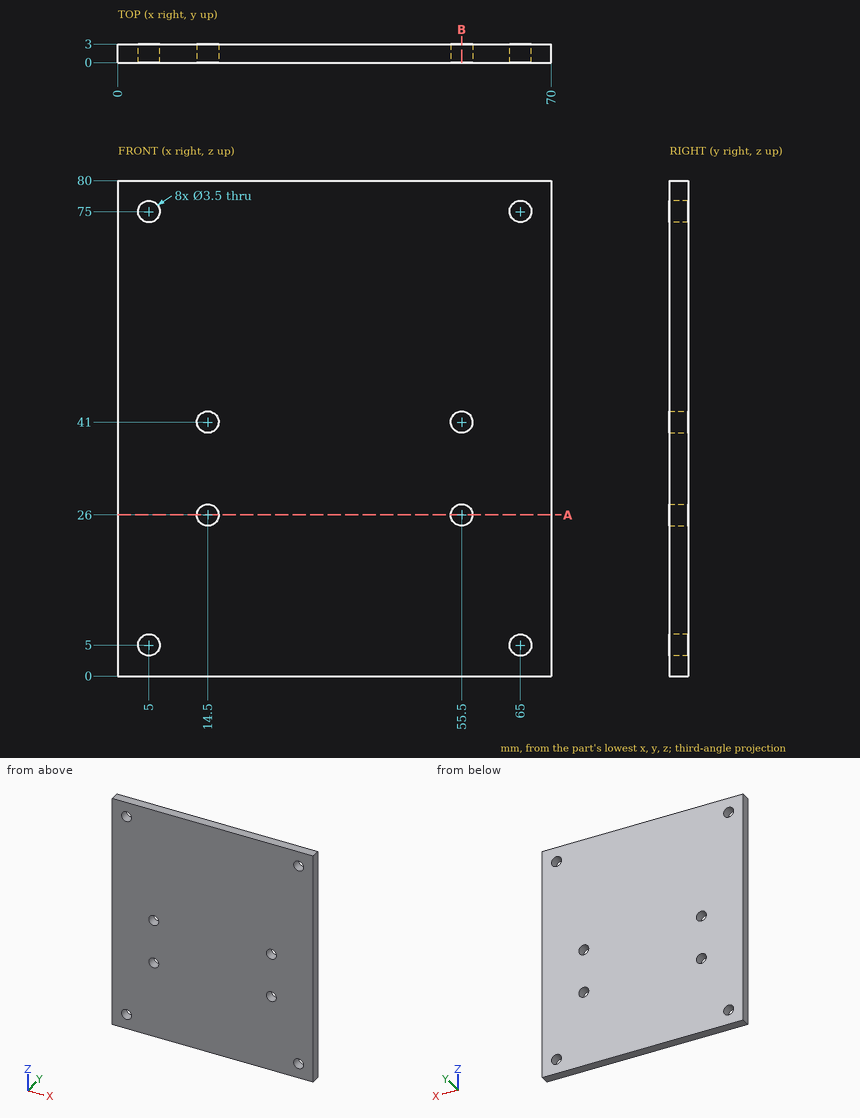
Drawing for the job (mm, zero at the part's lowest x, y, z). Round coordinates to 2 decimals unless told otherwise and drop trailing zeros. Write each loop counter-clockwise with the first axis right and the second up, starting at its lowest first coordinate (ties: lowest second). Pieces come first, ordered by that corner, then holes. Notation, with made-up numbers: M 84.5,47 L 128.5,47 A22 cw 128.5,58 Z; hole C 47.5,-39 d2. An arc over 180 degrees is marked long. One line per question, with ' | ' between items.
1. Cut at A-A on z = 26. Write the cut outline in (x, y).
Working result:
outline: M 0,0 L 12.75,0 L 12.75,3 L 0,3 Z; M 16.25,0 L 53.75,0 L 53.75,3 L 16.25,3 Z; M 57.25,0 L 70,0 L 70,3 L 57.25,3 Z
2. Probe L1, parallel to Z at x = 65, y = 2.3; L2, parallel to X at y = 1.35, z = 75; L3, parallel to X at y = 2.25, z = 41. List the from-to ranges inside material, lowest first. Write a range as from..to.
Working result:
L1: 0..3.25, 6.75..73.25, 76.75..80 | L2: 0..3.25, 6.75..63.25, 66.75..70 | L3: 0..12.75, 16.25..53.75, 57.25..70
3. Pin check, flat tip, straight feed: pin 1 Ø3 at (x, z) = (14.5, 41) entering from -Y. Stop position of the tip, or through.
Working result:
pin 1: through
4. Cut at B-B on x = 55.5. Write the cut outline in (y, z), and give its area (3 significant figures).
Working result:
outline: M 0,0 L 3,0 L 3,24.25 L 0,24.25 Z; M 0,27.75 L 3,27.75 L 3,39.25 L 0,39.25 Z; M 0,42.75 L 3,42.75 L 3,80 L 0,80 Z | area: 219 mm2
